Source: CAD feature listing. Evaluate the final solid. Frame: model axes, mm. Give positions to 0.01 mm unless a question says otherwise; leave off trailing zeros. Loops run counter-clockwise (first coordinate to the right, second up) from the corner with the lowest first, then second, coordinate; pieces in that order, holes last.
```python
from build123d import *

# Parameters (mm, degrees)
SKETCH1_W                      = 16.002
SKETCH1_H                      = 11.3284
BOSS_EXTRUDE1_DEPTH            = 76.2
F_9_0_196_DIAMETER_HOLE1_D     = 4.9784
F_9_0_196_DIAMETER_HOLE1_DEPTH = 15.24
F_9_0_196_DIAMETER_HOLE1_TIP   = 1.495662253
F_9_0_196_DIAMETER_HOLE2_D     = 4.9784
F_9_0_196_DIAMETER_HOLE2_DEPTH = 15.24
F_9_0_196_DIAMETER_HOLE2_TIP   = 1.495662253
SKETCH9_W                      = 9.652
SKETCH9_H                      = 3.302
CUT_EXTRUDE1_DEPTH             = 76.2


with BuildPart() as part:
    # Sketch1 → Boss-Extrude1 (new body)
    with BuildSketch(Plane(origin=(0, 0, 0), x_dir=(1, 0, 0), z_dir=(0, 1, 0))):
        Rectangle(SKETCH1_W, SKETCH1_H)
    extrude(amount=BOSS_EXTRUDE1_DEPTH)

    # #9 (0.196) Diameter Hole1
    with Locations(Plane(origin=(0, 76.2, 0), x_dir=(1, 0, 0), z_dir=(0, 1, 0))):
        with Locations((0, 0)):
            Hole(F_9_0_196_DIAMETER_HOLE1_D / 2, depth=F_9_0_196_DIAMETER_HOLE1_DEPTH)
            with Locations((0, 0, -(F_9_0_196_DIAMETER_HOLE1_DEPTH + F_9_0_196_DIAMETER_HOLE1_TIP / 2))):  # 118° drill point
                Cone(0, F_9_0_196_DIAMETER_HOLE1_D / 2, F_9_0_196_DIAMETER_HOLE1_TIP, mode=Mode.SUBTRACT)

    # #9 (0.196) Diameter Hole2
    with Locations(Plane(origin=(0, 0, 0), x_dir=(-1, 0, 0), z_dir=(0, -1, 0))):
        with Locations((0, 0)):
            Hole(F_9_0_196_DIAMETER_HOLE2_D / 2, depth=F_9_0_196_DIAMETER_HOLE2_DEPTH)
            with Locations((0, 0, -(F_9_0_196_DIAMETER_HOLE2_DEPTH + F_9_0_196_DIAMETER_HOLE2_TIP / 2))):  # 118° drill point
                Cone(0, F_9_0_196_DIAMETER_HOLE2_D / 2, F_9_0_196_DIAMETER_HOLE2_TIP, mode=Mode.SUBTRACT)

    # Sketch9 → Cut-Extrude1 (cut)
    with BuildSketch(Plane(origin=(0, 0, -5.6642), x_dir=(-1, 0, 0), z_dir=(0, 0, -1))):
        with Locations((0, 8.001)):
            Rectangle(SKETCH9_W, SKETCH9_H)
        with Locations((0, 68.199)):
            Rectangle(SKETCH9_W, SKETCH9_H)
    extrude(amount=-CUT_EXTRUDE1_DEPTH, mode=Mode.SUBTRACT)


solid = part.part
```
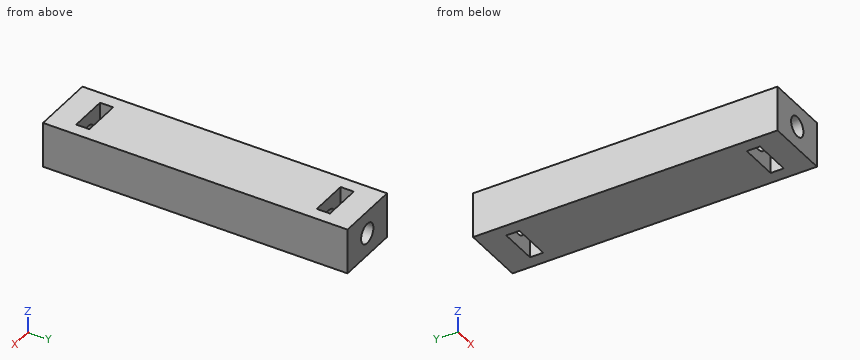
(1) Section B-B, the plane x = -4. Return the cut outline in (y, z), then the cut area to 3 significant figures.
A:
outline: (0, -5.66) - (6.35, -5.66) - (6.35, 5.66) - (0, 5.66) - close; (9.65, -5.66) - (66.55, -5.66) - (66.55, 5.66) - (9.65, 5.66) - close; (69.85, -5.66) - (76.2, -5.66) - (76.2, 5.66) - (69.85, 5.66) - close
area: 788 mm2
(2) Section C-C, the plane z = 3.75. Return the cut outline in (x, y).
A:
outline: (-8, 0) - (8, 0) - (8, 76.2) - (-8, 76.2) - close; hole (-4.83, 6.35) - (4.83, 6.35) - (4.83, 9.65) - (-4.83, 9.65) - close; hole (-4.83, 66.55) - (4.83, 66.55) - (4.83, 69.85) - (-4.83, 69.85) - close
(3) First-contact query: pin 1 (3 mm diameter, centred on x = 0, z = 0, fed in from +Y); pin 2 (4.5 mm diameter, centred on x = 0, z = 0, fed in from -Y). Flat tips, straight axial feed; report the tip coordinate or a pass-through.
A:
pin 1: stops at y = 60.37
pin 2: stops at y = 15.38
(4) Section A-A, the plane y = 68.5. Return the cut outline in (x, z), then the cut area to 3 significant figures.
A:
outline: (-8, -5.66) - (-4.83, -5.66) - (-4.83, 5.66) - (-8, 5.66) - close; (4.83, -5.66) - (8, -5.66) - (8, 5.66) - (4.83, 5.66) - close
area: 71.9 mm2
(5) Ray query, line 1 along Y through (x, z) = (4.75, -0.5); line 2 along X through (y, z) = (9.5, 2.5); line 3 along Z through (x, y) = (0, 64.7). Return the intervals inside material, ascending.
A:
line 1: y = 0 to 6.35, 9.65 to 66.55, 69.85 to 76.2
line 2: x = -8 to -4.83, 4.83 to 8
line 3: z = -5.66 to -2.49, 2.49 to 5.66
(6) Section D-D, the plane y = 13.5. Return the cut outline in (x, z), then the cut area to 3 significant figures.
A:
outline: (-8, -5.66) - (8, -5.66) - (8, 5.66) - (-8, 5.66) - close; hole circle Ø4.98 at (0, 0)
area: 162 mm2
